```python
from build123d import *

# Parameters (mm, degrees)
BOSS_EXTRUDE1_DEPTH      = 1.5
F_4_0_4_DIAMETER_HOLE1_D = 4
F_7_0_7_DIAMETER_HOLE1_D = 7
F_12_0MM_DOWEL_HOLE1_D   = 12


with BuildPart() as part:
    # Sketch1 → Boss-Extrude1 (new body)
    with BuildSketch(Plane.XY):
        with BuildLine():
            Line((50, 0), (310, 0))
            ThreePointArc((310, 0), (345.355339059, 14.644660941), (360, 50))
            Line((360, 50), (360, 310))
            ThreePointArc((360, 310), (345.355339059, 345.355339059), (310, 360))
            Line((310, 360), (50, 360))
            ThreePointArc((50, 360), (14.644660941, 345.355339059), (0, 310))
            Line((0, 310), (0, 50))
            ThreePointArc((0, 50), (14.644660941, 14.644660941), (50, 0))
        make_face()
    extrude(amount=BOSS_EXTRUDE1_DEPTH)

    # Ø4.0 (4) Diameter Hole1 (through all)
    with Locations(Plane(origin=(135, 210, 1.5), x_dir=(1, 0, 0), z_dir=(0, 0, 1))):
        with Locations((0, 0), (90, 0), (90, -60), (0, -60)):
            Hole(F_4_0_4_DIAMETER_HOLE1_D / 2)

    # Ø7.0 (7) Diameter Hole1 (through all)
    with Locations(Plane(origin=(152.5, 280, 1.5), x_dir=(1, 0, 0), z_dir=(0, 0, 1))):
        with Locations((0, 0), (55, 0)):
            Hole(F_7_0_7_DIAMETER_HOLE1_D / 2)

    # Ø12.0mm Dowel Hole1 (through all)
    with Locations(Plane(origin=(140, 235, 1.5), x_dir=(1, 0, 0), z_dir=(0, 0, 1))):
        with Locations((0, 0), (80, 0), (0, -110), (80, -110)):
            Hole(F_12_0MM_DOWEL_HOLE1_D / 2)


solid = part.part
```
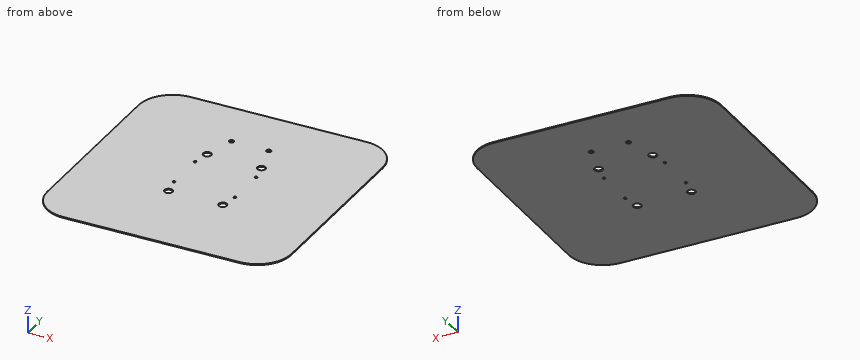
For this review, take the finished solid that the model builds, in its own axes (mm). Give positions to 0.01 mm unless a question says otherwise; leave off trailing zeros. Write each loop counter-clockwise with the first axis right and the second up, starting at its lowest first coordinate (ties: lowest second). Pieces come first, ordered by that corner, then holes. Notation, with made-up numbers: M 46,49.25 L 89,49.25 A24 ccw 89,87.25 Z; hole C -19,62 d9. An arc over 180 degrees is marked long. Answer as CSV lines item,"result".
1. Consider section A-A, the plane y = 235. Write out the cut boundary in (x, z), then the cut area to 3 significant figures.
Findings:
outline,"M 0,0 L 134,0 L 134,1.5 L 0,1.5 Z; M 146,0 L 214,0 L 214,1.5 L 146,1.5 Z; M 226,0 L 360,0 L 360,1.5 L 226,1.5 Z"
area,"504 mm2"
2. Consider section C-C, the plane x = 336.5. Write out the cut boundary in (y, z), then the cut area to 3 significant figures.
Findings:
outline,"M 7.6,0 L 352.4,0 L 352.4,1.5 L 7.6,1.5 Z"
area,"517 mm2"
3. Consider section B-B, the plane z = 0.5. Count the separate pieces of the cut face and the enclosed holes in it, then the cut area to 3 significant figures.
Findings:
separate pieces,"1"
enclosed holes,"10"
area,"127,000 mm2"
4. For pin 1 (2 mm diameter, centred on x = 221, y = 42.5, fed in from -Z), flat-tipped, find the tip position at first contact; note if it passes through.
Findings:
pin 1,"stops at z = 0"
5. Wall thickness on line 1 (Y direction, x = 139, z = 1.3); line 2 (X direction, y = 210, z = 0.9); line 3 (Y direction, x = 220, z = 0.35): over which ranges is each line inside the solid? List them lowest first.
Findings:
line 1,"y = 0 to 119.08, 130.92 to 229.08, 240.92 to 360"
line 2,"x = 0 to 133, 137 to 223, 227 to 360"
line 3,"y = 0 to 119, 131 to 229, 241 to 360"
